The model under review builds one solid part; all positions refer to its coordinate system, in mm. A direction names the side the tool comes from. Give positions to 0.01 mm unless a question says otherwise; leave off trailing zeros. Loops run counter-clockwise (first coordinate to the right, second up) from the corner with the lowest first, then second, coordinate; pieces in that order, holes last. Notation, with made-up numbers: M 12.25,-3 L 33.25,-3 A25 cw 33.25,15 Z; hole C 12,88 d4. An arc over 180 degrees is marked long. Write item = value, one per line. Start each with the question number.
1. For faces 4 (the face through (17.717, 3.131, 11.731)), 5 (the face through (15.73, 3.13, 14.73)), 6 (the face through (5.41, 3.131, 9.404)), list the 3-axis set-ups (+Z, -Z, +X, -X, +Y, -Y) from which the entire face can be reached by the end or side of a thin tool; tool diameter is ignored.
2. For pin 1 (3 mm diameter, centred on x = 8, y = 2.5, fed in from +Z); pin 2 (1 mm diameter, centred on x = 10, y = 2, fed in from +Z); pin 3 (1 mm diameter, centred on x = 11, y = 2.5, fed in from +Z), all flat-tipped, find the tip position at first contact; note any pin that passes through.
3. We need section D-D on x = 15.5. Give the boundary of the cut face in (y, z).
4. We need section A-A on x = 7.25. Give the boundary of the cut face in (y, z).
5. Wall thickness on line 1 along Z through (x, y) = (16.5, 1); line 2 along X through (y, z) = (4.5, 4.25); line 3 along X through (y, z) = (2, 14.75): over which ranges is each line inside the solid? List them lowest first. Write a range as from..to.
6. We need section C-C on z = 7.75. Give the boundary of the cut face in (x, y), then the cut area to 3 significant figures.
7. We need section B-B on z = 12. Give the boundary of the cut face in (x, y), then the cut area to 3 significant figures.
8. Draft analysis for pull direction X (two halves, no side actions). For faces 1 (the face through (16.47, 3.13, 5.87)), 2 (the face through (5.686, 3.131, 11.84)), 3 (the face through (8.67, 3.13, 4.38)), state which applies: pulls with the +X half, pulls with the -X half, needs draft (parallel to the pull), parting line crosses it, or undercut.
from build123d import *

# Parameters (mm, degrees)
BOSS_EXTRUDE1_DEPTH = 6.35


with BuildPart() as part:
    # Sketch1 → Boss-Extrude1 (new body)
    with BuildSketch(Plane(origin=(0, 0, 0), x_dir=(1, 0, 0), z_dir=(0, 1, 0))):
        with BuildLine():
            ThreePointArc((9.101190716, -14.617505223), (8.787991723, -15.525786229), (8.834558587, -16.485421328))
            ThreePointArc((8.834558587, -16.485421328), (9.005966344, -16.556955762), (9.179175886, -16.624009833))
            ThreePointArc((9.179175886, -16.624009833), (9.877166505, -15.963799948), (10.280004433, -15.09156741))
            ThreePointArc((10.280004433, -15.09156741), (10.682561911, -15.183548614), (11.091017353, -15.244188674))
            ThreePointArc((11.091017353, -15.244188674), (11.149243306, -16.203186971), (11.559501933, -17.07195383))
            ThreePointArc((11.559501933, -17.07195383), (11.745237093, -17.072448121), (11.930922326, -17.068113582))
            ThreePointArc((11.930922326, -17.068113582), (12.323130188, -16.191049737), (12.361514963, -15.231052547))
            ThreePointArc((12.361514963, -15.231052547), (12.768629261, -15.161980021), (13.16919883, -15.061695001))
            ThreePointArc((13.16919883, -15.061695001), (13.589985356, -15.925411791), (14.301477588, -16.571048531))
            ThreePointArc((14.301477588, -16.571048531), (14.473263658, -16.500427428), (14.643155688, -16.425364174))
            ThreePointArc((14.643155688, -16.425364174), (14.669870701, -15.464971388), (14.33795859, -14.563360415))
            ThreePointArc((14.33795859, -14.563360415), (14.687650245, -14.343749825), (15.019350856, -14.09780721))
            ThreePointArc((15.019350856, -14.09780721), (15.738637021, -14.734749443), (16.643044616, -15.058963723))
            ThreePointArc((16.643044616, -15.058963723), (16.774728723, -14.927978648), (16.902963029, -14.793614379))
            ThreePointArc((16.902963029, -14.793614379), (16.560118075, -13.896103748), (15.908439687, -13.19014109))
            ThreePointArc((15.908439687, -13.19014109), (16.147471316, -12.853426158), (16.359804557, -12.499268481))
            ThreePointArc((16.359804557, -12.499268481), (17.268085563, -12.812467475), (18.227720662, -12.76590061))
            ThreePointArc((18.227720662, -12.76590061), (18.299255096, -12.594492854), (18.366309167, -12.421283311))
            ThreePointArc((18.366309167, -12.421283311), (17.706099281, -11.723292693), (16.833866744, -11.320454765))
            ThreePointArc((16.833866744, -11.320454765), (16.925847948, -10.917897287), (16.986488008, -10.509441845))
            ThreePointArc((16.986488008, -10.509441845), (17.945486305, -10.451215891), (18.814253164, -10.040957265))
            ThreePointArc((18.814253164, -10.040957265), (18.814747455, -9.855222104), (18.810412916, -9.669536871))
            ThreePointArc((18.810412916, -9.669536871), (17.93334907, -9.27732901), (16.973351881, -9.238944234))
            ThreePointArc((16.973351881, -9.238944234), (16.904279354, -8.831829937), (16.803994334, -8.431260368))
            ThreePointArc((16.803994334, -8.431260368), (17.667711125, -8.010473841), (18.313347865, -7.29898161))
            ThreePointArc((18.313347865, -7.29898161), (18.242726762, -7.12719554), (18.167663508, -6.957303509))
            ThreePointArc((18.167663508, -6.957303509), (17.207270722, -6.930588496), (16.305659749, -7.262500608))
            ThreePointArc((16.305659749, -7.262500608), (16.086049159, -6.912808952), (15.840106544, -6.581108342))
            ThreePointArc((15.840106544, -6.581108342), (16.477048777, -5.861822176), (16.801263057, -4.957414582))
            ThreePointArc((16.801263057, -4.957414582), (16.670277982, -4.825730474), (16.535913713, -4.697496168))
            ThreePointArc((16.535913713, -4.697496168), (15.638403082, -5.040341123), (14.932440424, -5.69201951))
            ThreePointArc((14.932440424, -5.69201951), (14.595725492, -5.452987882), (14.241567815, -5.240654641))
            ThreePointArc((14.241567815, -5.240654641), (14.554766809, -4.332373635), (14.508199944, -3.372738536))
            ThreePointArc((14.508199944, -3.372738536), (14.336792188, -3.301204102), (14.163582645, -3.234150031))
            ThreePointArc((14.163582645, -3.234150031), (13.465592027, -3.894359916), (13.062754098, -4.766592453))
            ThreePointArc((13.062754098, -4.766592453), (12.66019662, -4.67461125), (12.251741179, -4.61397119))
            ThreePointArc((12.251741179, -4.61397119), (12.193515225, -3.654972893), (11.783256599, -2.786206034))
            ThreePointArc((11.783256599, -2.786206034), (11.597521438, -2.785711743), (11.411836205, -2.790046281))
            ThreePointArc((11.411836205, -2.790046281), (11.019628344, -3.667110127), (10.981243568, -4.627107317))
            ThreePointArc((10.981243568, -4.627107317), (10.574129271, -4.696179843), (10.173559702, -4.796464863))
            ThreePointArc((10.173559702, -4.796464863), (9.752773175, -3.932748072), (9.041280943, -3.287111332))
            ThreePointArc((9.041280943, -3.287111332), (8.869494873, -3.357732436), (8.699602843, -3.43279569))
            ThreePointArc((8.699602843, -3.43279569), (8.67288783, -4.393188476), (9.004799941, -5.294799449))
            ThreePointArc((9.004799941, -5.294799449), (8.655108286, -5.514410038), (8.323407676, -5.760352653))
            ThreePointArc((8.323407676, -5.760352653), (7.60412151, -5.123410421), (6.699713916, -4.799196141))
            ThreePointArc((6.699713916, -4.799196141), (6.568029808, -4.930181216), (6.439795502, -5.064545485))
            ThreePointArc((6.439795502, -5.064545485), (6.782640457, -5.962056116), (7.434318844, -6.668018774))
            ThreePointArc((7.434318844, -6.668018774), (7.195287216, -7.004733706), (6.982953975, -7.358891382))
            ThreePointArc((6.982953975, -7.358891382), (6.074672968, -7.045692389), (5.11503787, -7.092259254))
            ThreePointArc((5.11503787, -7.092259254), (5.043503436, -7.26366701), (4.976449365, -7.436876552))
            ThreePointArc((4.976449365, -7.436876552), (5.63665925, -8.134867171), (6.508891787, -8.537705099))
            ThreePointArc((6.508891787, -8.537705099), (6.416910584, -8.940262577), (6.356270524, -9.348718019))
            ThreePointArc((6.356270524, -9.348718019), (5.397272226, -9.406943972), (4.528505368, -9.817202599))
            ThreePointArc((4.528505368, -9.817202599), (4.528011077, -10.002937759), (4.532345615, -10.188622993))
            ThreePointArc((4.532345615, -10.188622993), (5.409409461, -10.580830854), (6.369406651, -10.61921563))
            ThreePointArc((6.369406651, -10.61921563), (6.438479177, -11.026329927), (6.538764197, -11.426899496))
            ThreePointArc((6.538764197, -11.426899496), (5.675047406, -11.847686023), (5.029410666, -12.559178254))
            ThreePointArc((5.029410666, -12.559178254), (5.10003177, -12.730964324), (5.175095023, -12.900856355))
            ThreePointArc((5.175095023, -12.900856355), (6.13548781, -12.927571367), (7.037098782, -12.595659256))
            ThreePointArc((7.037098782, -12.595659256), (7.256709372, -12.945350911), (7.502651987, -13.277051522))
            ThreePointArc((7.502651987, -13.277051522), (6.865709755, -13.996337688), (6.541495474, -14.900745282))
            ThreePointArc((6.541495474, -14.900745282), (6.672480549, -15.032429389), (6.806844819, -15.160663695))
            ThreePointArc((6.806844819, -15.160663695), (7.70435545, -14.817818741), (8.410318108, -14.166140353))
            ThreePointArc((8.410318108, -14.166140353), (8.74703304, -14.405171982), (9.101190716, -14.617505223))
        make_face()
        with BuildLine():
            Line((9.961117692, -7.254078932), (13.381640839, -7.254078932))
            ThreePointArc((13.381640839, -7.254078932), (11.671379266, -13.104079932), (9.961117692, -7.254078932))
        make_face(mode=Mode.SUBTRACT)
    extrude(amount=BOSS_EXTRUDE1_DEPTH)


solid = part.part
Final values:
q1.face_4 = +X, +Y, -Y
q1.face_5 = +Z, +Y, -Y
q1.face_6 = +Y, -Y
q2.pin_1 = 16.62
q2.pin_2 = 16.38
q2.pin_3 = 16.99
q3.outline = M 0,5.13 L 6.35,5.13 L 6.35,14.57 L 0,14.57 Z
q4.outline = M 0,4.95 L 6.35,4.95 L 6.35,6.52 L 0,6.52 Z; M 0,6.92 L 6.35,6.92 L 6.35,12.94 L 0,12.94 Z; M 0,13.5 L 6.35,13.5 L 6.35,15.04 L 0,15.04 Z
q5.line_1 = 4.7..5.82, 7.16..12.57, 13.8..15.03
q5.line_2 = 8.65..9.96, 10.95..12.27, 13.25..14.57
q5.line_3 = 6.57..7.81, 9.03..14.44, 15.76..16.89
q6.outline = M 5.21,0 L 9.36,0 L 9.36,6.35 L 5.21,6.35 Z; M 13.98,0 L 17.96,0 L 17.96,6.35 L 13.98,6.35 Z
q6.area = 51.6 mm²
q7.outline = M 5.49,0 L 9.26,0 L 9.26,6.35 L 5.49,6.35 Z; M 14.08,0 L 18.03,0 L 18.03,6.35 L 14.08,6.35 Z
q7.area = 49.1 mm²
q8.face_1 = pulls with the +X half
q8.face_2 = pulls with the -X half
q8.face_3 = undercut
